Solid Edge part; units mm, degrees
sketch "Sketch1" plane through (0, 0, 0) normal (0, 0, 1) x (1, 0, 0)
  line L0 (10, -18.75) -> (-10, -18.75)
  line L1 (-10, -18.75) -> (-10, 18.75)
  line L2 (-10, 18.75) -> (10, 18.75)
  line L3 (10, 18.75) -> (10, -18.75)
extrude "Protrusion1" add sketch "Sketch1" along normal blind 40
hole "Bohrung_6" at (0, -11.25, 40) direction (0, 0, -1) diameter 4.917 depth 15 thread major 6 thread length 10
fillet "Verrundung_1" radius 1 4 edges at (-10, 0, 40) (10, 0, 40) (-10, 0, 0) (10, 0, 0)
hole "Bohrung_4" at (0, -18.75, 22) direction (0, 1, 0) diameter 6.5 end through all
hole "Hole1" at (0, -18.75, 7) direction (0, 1, 0) diameter 6.5 end through all
Can you work these out from the model? Positions are in its coordinate system, mm. A direction names the side the tool comes from. Round coordinates to 2 decimals unless told otherwise and drop trailing zeros. Loops run counter-clockwise (first coordinate to the right, second up) from the corner with the lowest first, then second, coordinate; pieces in that order, holes last. Notation, with made-up numbers: (72.5, 69) - (109.5, 69) arc R19 cw to (109.5, 73) - close; hole circle Ø2 at (70, 38.5). An arc over 180 degrees is marked (long way). Use CSV: the item, a comma, the result in double quotes. Start each with the question number.
1) If we section it at D-D on z = 29.5: Write out the boundary of the cut face in (x, y).
2) If we section it at B-B on y = -11.25: Write out the boundary of the cut face in (x, z), plus the area to 3 significant figures.
3) We'd pull the mould along Z, two halves only. Please class faces 3 (the cylindrical face through (0.98, -0.26, 18.9)), 4 (the cylindrical face through (-0.108, -8.794, 32.395)), 5 (the cylindrical face through (0.143, -0.262, 10.247)), 6 (the cylindrical face through (-9.715, 0.262, 39.699)): released by +Z, released by -Z, zero draft, split by the parting line, or undercut.
4) For pin 1 Ø6.5 at (x, y) = (0, -11.25) entering from +Z, with a flat end and sliding along its axis, tell me the tip position at first contact or that it passes through.
5) For faces 1 (the flat face through (2, -11, 25)), 2 (the flat face through (0, 0, 0)), which set-ups out of +Z, -Z, +X, -X, +Y, -Y let a thin tool reach every point of the face, with its end or its side?
6) Please list where these lines run through material, in increasing order: probe 1 along Z at (x, y) = (-2.5, -15); probe 2 along X at (y, z) = (8.5, 7); probe 3 along Z at (x, y) = (3, -5). Write a range as [from, to].
7) If we section it at C-C on z = 7: Write out the boundary of the cut face in (x, y).
8) If we section it at A-A on x = 0: Write out the boundary of the cut face in (y, z).
Geometry results:
1,outline,"(-10, -18.75) - (10, -18.75) - (10, 18.75) - (-10, 18.75) - close; hole circle Ø4.92 at (0, -11.25)"
2,outline,"(-10, 1) arc R1 ccw to (-9, 0) - (9, 0) arc R1 ccw to (10, 1) - (10, 39) arc R1 ccw to (9, 40) - (2.46, 40) - (2.46, 25) - (1.25, 25) arc R3.25 cw (long way) to (-1.25, 25) - (-2.46, 25) - (-2.46, 40) - (-9, 40) arc R1 ccw to (-10, 39) - close; hole circle Ø6.5 at (0, 7)"
2,area,"659 mm2"
3,face 3,"undercut"
3,face 4,"zero draft"
3,face 5,"undercut"
3,face 6,"released by +Z"
4,pin 1,"stops at z = 40"
5,face 1,"+Z"
5,face 2,"-Z, +X, -X, +Y, -Y"
6,probe 1,"z = [0, 4.92], [9.08, 19.92], [24.08, 40]"
6,probe 2,"x = [-10, -3.25], [3.25, 10]"
6,probe 3,"z = [0, 5.75], [8.25, 20.75], [23.25, 40]"
7,outline,"(-10, -18.75) - (-3.25, -18.75) - (-3.25, 18.75) - (-10, 18.75) - close; (3.25, -18.75) - (10, -18.75) - (10, 18.75) - (3.25, 18.75) - close"
8,outline,"(-18.75, 0) - (18.75, 0) - (18.75, 3.75) - (-18.75, 3.75) - close; (-18.75, 10.25) - (18.75, 10.25) - (18.75, 18.75) - (-18.75, 18.75) - close; (-18.75, 25.25) - (-13.71, 25.25) - (-13.71, 40) - (-18.75, 40) - close; (-8.79, 25.25) - (18.75, 25.25) - (18.75, 40) - (-8.79, 40) - close"
